```python
from build123d import *

# Parameters (mm, degrees)
BOX008_W          = 26
BOX008_H          = 190
BOX008_DEPTH      = 32
CYLINDER011_R     = 5
CYLINDER011_DEPTH = 16
CYLINDER010_R     = 5
CYLINDER010_DEPTH = 16
BOX006_W          = 82
BOX006_H          = 190
BOX006_DEPTH      = 8
BOX007_W          = 26
BOX007_H          = 190
BOX007_DEPTH      = 32


with BuildPart() as box008:
    # Box008 → Box008 (new body)
    with BuildSketch(Plane.XY.offset(8)):
        with Locations((13, 95)):
            Rectangle(BOX008_W, BOX008_H)
    extrude(amount=BOX008_DEPTH)


with BuildPart() as cylinder011:
    # Cylinder011 → Cylinder011 (new body)
    with BuildSketch(Plane(origin=(41, 167, -4), x_dir=(1, 0, 0), z_dir=(0, 0, 1))):
        Circle(CYLINDER011_R)
    extrude(amount=CYLINDER011_DEPTH)


with BuildPart() as cylinder010:
    # Cylinder010 → Cylinder010 (new body)
    with BuildSketch(Plane(origin=(41, 43, -4), x_dir=(1, 0, 0), z_dir=(0, 0, 1))):
        Circle(CYLINDER010_R)
    extrude(amount=CYLINDER010_DEPTH)


with BuildPart() as suelo_taladrado:
    # Box006 → Box006 (new body)
    with BuildSketch(Plane.XY):
        with Locations((41, 95)):
            Rectangle(BOX006_W, BOX006_H)
    extrude(amount=BOX006_DEPTH)

    # Cut002: cut Cylinder010
    add(cylinder010.part, mode=Mode.SUBTRACT)

    # Cut003: cut Cylinder011
    add(cylinder011.part, mode=Mode.SUBTRACT)


with BuildPart() as suelo_final:
    # Box007 → Box007 (new body)
    with BuildSketch(Plane(origin=(56, 0, 8), x_dir=(1, 0, 0), z_dir=(0, 0, 1))):
        with Locations((13, 95)):
            Rectangle(BOX007_W, BOX007_H)
    extrude(amount=BOX007_DEPTH)

    # Fusion003: union Box008, Suelo taladrado
    add(box008.part)
    add(suelo_taladrado.part)


solid = suelo_final.part
```
Geometry: final body of the model. Coordinates: model frame, mm. A direction names the side the tool comes from. Coordinates: 2 decimals unless noted, no trailing zeros. Write each loop counter-clockwise with the first axis right and the second up, starting at its lowest first coordinate (ties: lowest second). Pieces come first, ordered by that corner, then holes. Notation, with made-up numbers: M -10,-37.75 L 5,-37.75 A23 ccw 5,-14.75 Z; hole C 29,-2.5 d11. An arc over 180 degrees is marked long. Answer as CSV lines item,"result". Start each with the question number.
Q1. Pin query (flat end, axial travel): P1, Ø15, axis at x = 35, y = 76, coming from the +Z side. Return the tip coordinate at first contact, or that it passes through.
Q2. Cut plane B-B on y = 43. Return the cut outline in (x, z).
Q3. Line query: line 1 (Y direction, x = 41, z = 5.5); line 2 (X direction, y = 135, z = 33); line 3 (X direction, y = 167, z = 3.25). Output: solid intervals per line, ascending. Write a range as from..to.
Q4. Mould query, pull axis Y, two halves, no side actions, for faces 3 (the cylindrical face through (37, 46, 4)), 4 (the flat face through (40, 0, 6)), 5 (the flat face through (69, 96, 40)). Classes: released by +Y, released by -Y, zero draft, split by the parting line, or undercut.
Q5. Cut plane C-C on z = 33. Return the cut outline in (x, y).
Q6. Reachability of faces 1 (the cylindrical face through (40.349, 171.957, 3.944)), 2 (the flat face through (56, 94, 24)) from +Z, -Z, +X, -X, +Y, -Y: full face, straight path, thin tool, end or side. Return the list, or none.
Q7. Cut plane D-D on y = 177.5. Return the cut outline in (x, z), then the cut area to 3 significant figures.
Q8. Cut plane A-A on x = 41. Return the cut outline in (y, z), then the cut area to 3 significant figures.
Findings below:
1,P1,"stops at z = 8"
2,outline,"M 0,0 L 36,0 L 36,8 L 26,8 L 26,40 L 0,40 Z; M 46,0 L 82,0 L 82,40 L 56,40 L 56,8 L 46,8 Z"
3,line 1,"y = 0..38, 48..162, 172..190"
3,line 2,"x = 0..26, 56..82"
3,line 3,"x = 0..36, 46..82"
4,face 3,"undercut"
4,face 4,"released by -Y"
4,face 5,"zero draft"
5,outline,"M 0,0 L 26,0 L 26,190 L 0,190 Z; M 56,0 L 82,0 L 82,190 L 56,190 Z"
6,face 1,"+Z, -Z"
6,face 2,"+Z, +Y, -Y"
7,outline,"M 0,0 L 82,0 L 82,40 L 56,40 L 56,8 L 26,8 L 26,40 L 0,40 Z"
7,area,"2,320 mm2"
8,outline,"M 0,0 L 38,0 L 38,8 L 0,8 Z; M 48,0 L 162,0 L 162,8 L 48,8 Z; M 172,0 L 190,0 L 190,8 L 172,8 Z"
8,area,"1,360 mm2"
